```python
from build123d import *

# Parameters (mm, degrees)
SKETCH1_W                      = 56
SKETCH1_H                      = 51
BOSS_EXTRUDE1_DEPTH            = 17
SKETCH2_W                      = 56
SKETCH2_H                      = 51
SKETCH2_R                      = 8.9
BOSS_EXTRUDE2_DEPTH            = 8.5
CBORE_FOR_M3_SHCS1_D           = 3.6
CBORE_FOR_M3_SHCS1_CBORE_D     = 6.5
CBORE_FOR_M3_SHCS1_CBORE_DEPTH = 23
FILLET3_R                      = 3
M2_5X0_45_TAPPED_HOLE1_D       = 2.05
M2_5X0_45_TAPPED_HOLE1_DEPTH   = 10
M2_5X0_45_TAPPED_HOLE1_TIP     = 0.615882135
FILLET4_R                      = 3


with BuildPart() as part:
    # Sketch1 → Boss-Extrude1 (new body)
    with BuildSketch(Plane(origin=(0, 0, 0), x_dir=(1, 0, 0), z_dir=(0, 1, 0))):
        Rectangle(SKETCH1_W, SKETCH1_H)
        Polygon((15, -15), (-15, -15), (-15, -7.5), (-20, -7.5), (-20, 7.5), (-15, 7.5), (-15, 15), (15, 15), (15, 7.5), (20, 7.5), (20, -7.5), (15, -7.5), align=None, mode=Mode.SUBTRACT)
    extrude(amount=BOSS_EXTRUDE1_DEPTH)

    # Sketch2 → Boss-Extrude2 (add)
    with BuildSketch(Plane(origin=(0, 17, 0), x_dir=(1, 0, 0), z_dir=(0, 1, 0))):
        Rectangle(SKETCH2_W, SKETCH2_H)
        with Locations(Location((0, 0, 0), (0, 0, 270))):
            Circle(SKETCH2_R, mode=Mode.SUBTRACT)
    extrude(amount=BOSS_EXTRUDE2_DEPTH)

    # CBORE for M3 SHCS1 (through all)
    with Locations(Plane(origin=(0, 25.5, 0), x_dir=(1, 0, 0), z_dir=(0, 1, 0))):
        with Locations((-17.5, 17.5), (17.5, 17.5), (17.5, -17.5), (-17.5, -17.5)):
            CounterBoreHole(CBORE_FOR_M3_SHCS1_D / 2, CBORE_FOR_M3_SHCS1_CBORE_D / 2, CBORE_FOR_M3_SHCS1_CBORE_DEPTH)

    # Fillet3
    fillet3_edges = [part.edges().sort_by_distance(p)[0] for p in [
        (-28, 25.5, 0),
        (28, 25.5, 0),
    ]]
    fillet(fillet3_edges, radius=FILLET3_R)

    # M2.5x0.45 Tapped Hole1
    with Locations(Plane(origin=(0, 0, -25.5), x_dir=(-1, 0, 0), z_dir=(0, 0, -1))):
        with Locations((-23, 20.5), (23, 20.5), (-23, 5), (23, 5)):
            Hole(M2_5X0_45_TAPPED_HOLE1_D / 2, depth=M2_5X0_45_TAPPED_HOLE1_DEPTH)
            with Locations((0, 0, -(M2_5X0_45_TAPPED_HOLE1_DEPTH + M2_5X0_45_TAPPED_HOLE1_TIP / 2))):  # 118° drill point
                Cone(0, M2_5X0_45_TAPPED_HOLE1_D / 2, M2_5X0_45_TAPPED_HOLE1_TIP, mode=Mode.SUBTRACT)

    # Fillet4
    fillet4_edges = [part.edges().sort_by_distance(p)[0] for p in [
        (28, 11.25, 25.5),
        (-28, 11.25, 25.5),
        (-27.121320344, 24.621320344, 25.5),
        (27.121320344, 24.621320344, 25.5),
        (0, 25.5, 25.5),
    ]]
    fillet(fillet4_edges, radius=FILLET4_R)


solid = part.part
```
Check sheet for the modelled part. Datum: model origin and axes. Units: mm. A direction names the side the tool comes from. Give positions to 0.01 mm unless a question says otherwise; leave off trailing zeros. Write each loop counter-clockwise with the first axis right and the second up, starting at its lowest first coordinate (ties: lowest second). Pieces come first, ordered by that corner, then holes. Notation, with made-up numbers: (23, 4) - (40, 4) arc R32 cw to (40, 34) - close; hole circle Ø4 at (33, 88.5). An arc over 180 degrees is marked (long way). Answer as a JSON object with one key per item and string values. Group by question number.
1) Access from +Z, -Z, +X, -X, +Y, -Y to the whole of each face (thin tool, end or side, straight path). Record for faces 4 (the face through (-23.76, 21.19, -20.43)), 5 (the face through (15.105, 14.161, -19.697)), 6 (the face through (-20, 8, 0)).
2) Sectioned sample at C-C (z = 0). Record the cut outline in (x, y).
3) Sectioned sample at B-B (y = 11.5). Record the cut outline in (x, z), then the cut area to 3 significant figures.
4) Sectioned sample at D-D (x = 0). Record the cut outline in (y, z), then the cut area to 3 significant figures.
5) Thickness scan on probe 1 along Y at (x, z) = (-23, -20) (3 decimals); probe 2 along X at (y, z) = (20.5, -22.75) (3 decimals); probe 3 along Z at (x, y) = (17.5, 20.25). Record the ranges inside material, lowest first. Write a range as from..to.
6) Sectioned sample at A-A (x = -17.5). Record the cut outline in (y, z).
7) Release check for a two-part mould opening along Y. For faces 1 (the face through (27.1, 24.64, -1.84)), 2 (the face through (22.24, 21.19, -20.43)), 3 (the face through (17, 8, -7.5)) record: pulls with the +Y half, pulls with the -Y half, needs draft (parallel to the pull), parting line crosses it, or undercut.
8) Depth check by flat-ended pin: P1, Ø1.8, axis at x = 23, y = 20.5, coming from the -Z side; P2, Ø1, axis at x = -13.5, z = 0.5, coming from the -Y side; P3, Ø2, axis at x = -17, z = 18.5, coming from the +Y side; P4, Ø3, axis at x = -17.5, z = 17.5, coming from the +Y side. Enter the tip coordinate at first touch or a pass-through.
Geometry results:
{
 "1": {"face 4": "-Z", "face 5": "+Y", "face 6": "-Y"},
 "2": {"outline": "(-28, 0) - (-20, 0) - (-20, 17) - (-8.9, 17) - (-8.9, 25.5) - (-25, 25.5) arc R3 ccw to (-28, 22.5) - close; (8.9, 17) - (20, 17) - (20, 0) - (28, 0) - (28, 22.5) arc R3 ccw to (25, 25.5) - (8.9, 25.5) - close"},
 "3": {"outline": "(-28, -25.5) - (28, -25.5) - (28, 22.5) arc R3 ccw to (25, 25.5) - (-25, 25.5) arc R3 ccw to (-28, 22.5) - close; hole circle Ø6.5 at (-17.5, -17.5); hole circle Ø6.5 at (-17.5, 17.5); hole (-20, -7.5) - (-15, -7.5) - (-15, -15) - (15, -15) - (15, -7.5) - (20, -7.5) - (20, 7.5) - (15, 7.5) - (15, 15) - (-15, 15) - (-15, 7.5) - (-20, 7.5) - close; hole circle Ø6.5 at (17.5, -17.5); hole circle Ø6.5 at (17.5, 17.5)", "area": "1,670 mm^2"},
 "4": {"outline": "(0, -25.5) - (25.5, -25.5) - (25.5, -8.9) - (17, -8.9) - (17, -15) - (0, -15) - close; (0, 15) - (17, 15) - (17, 8.9) - (25.5, 8.9) - (25.5, 22.5) arc R3 ccw to (22.5, 25.5) - (0, 25.5) - close", "area": "637 mm^2"},
 "5": {"probe 1": "y = 0..3.975, 6.025..19.475, 21.525..25.5", "probe 2": "x = -28..-24.025, -21.975..21.975, 24.025..28", "probe 3": "z = -25.5..-20.75, -14.25..14.25, 20.75..25.5"},
 "6": {"outline": "(0, -25.5) - (25.5, -25.5) - (25.5, -20.75) - (2.5, -20.75) - (2.5, -19.3) - (0, -19.3) - close; (0, -15.7) - (2.5, -15.7) - (2.5, -14.25) - (25.5, -14.25) - (25.5, 14.25) - (2.5, 14.25) - (2.5, 15.7) - (0, 15.7) - (0, 7.5) - (17, 7.5) - (17, -7.5) - (0, -7.5) - close; (0, 19.3) - (2.5, 19.3) - (2.5, 20.75) - (25.5, 20.75) - (25.5, 22.5) arc R3 ccw to (22.5, 25.5) - (0, 25.5) - close"},
 "7": {"face 1": "pulls with the +Y half", "face 2": "undercut", "face 3": "needs draft"},
 "8": {"P1": "stops at z = -15.42", "P2": "stops at y = 17", "P3": "stops at y = 2.5", "P4": "passes through"}
}
